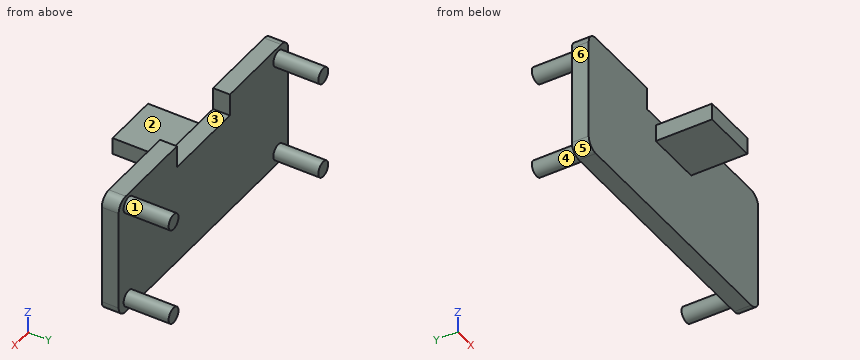
```python
from build123d import *

# Parameters (mm, degrees)
SKETCH1_W           = 48
SKETCH1_H           = 22
BOSS_EXTRUDE1_DEPTH = 3
SKETCH2_R           = 1.4
BOSS_EXTRUDE2_DEPTH = 8
SKETCH3_W           = 10
SKETCH3_H           = 3
BOSS_EXTRUDE3_DEPTH = 10
SKETCH4_W           = 15
SKETCH4_H           = 4
CUT_EXTRUDE1_DEPTH  = 10
FILLET1_R           = 2


with BuildPart() as part:
    # Sketch1 → Boss-Extrude1 (new body)
    with BuildSketch(Plane(origin=(0, 0, 0), x_dir=(1, 0, 0), z_dir=(0, 1, 0))):
        Rectangle(SKETCH1_W, SKETCH1_H)
    extrude(amount=BOSS_EXTRUDE1_DEPTH)

    # Sketch2 → Boss-Extrude2 (add)
    with BuildSketch(Plane(origin=(0, 3, 0), x_dir=(1, 0, 0), z_dir=(0, 1, 0))):
        with Locations((-21.2, 8.899999974)):
            Circle(SKETCH2_R)
        with Locations((-21.2, -8.899999974)):
            Circle(SKETCH2_R)
        with Locations((21.2, 8.899999974)):
            Circle(SKETCH2_R)
        with Locations((21.2, -8.899999974)):
            Circle(SKETCH2_R)
    extrude(amount=BOSS_EXTRUDE2_DEPTH)

    # Sketch3 → Boss-Extrude3 (add)
    with BuildSketch(Plane.XZ):
        with Locations((0, 4.044761195)):
            Rectangle(SKETCH3_W, SKETCH3_H)
    extrude(amount=BOSS_EXTRUDE3_DEPTH)

    # Sketch4 → Cut-Extrude1 (cut)
    with BuildSketch(Plane.XZ):
        with Locations((0, 9)):
            Rectangle(SKETCH4_W, SKETCH4_H)
    extrude(amount=-CUT_EXTRUDE1_DEPTH, mode=Mode.SUBTRACT)

    # Fillet1
    fillet1_edges = [part.edges().sort_by_distance(p)[0] for p in [
        (24, 1.5, 11),
        (-24, 1.5, 11),
        (-24, 1.5, -11),
        (24, 1.5, -11),
    ]]
    fillet(fillet1_edges, radius=FILLET1_R)


solid = part.part
```
Design review of the part built by this model. Coordinates are the model's own, in mm. Face numbers are marked on the shaded views. A direction names the side the tool comes from. Round coordinates to 2 decimals unless told otherwise and drop trailing zeros. Write each loop counter-clockwise with the first axis right and the second up, starting at its lowest first coordinate (ties: lowest second). Pieces come first, ordered by that corner, then holes.
Item 1: We need section A-A on x = 21.2. Write out the cut boundary in (y, z), and give its area (3 significant figures).
Item 2: We need section C-C on z = -8.25. Write out the cut boundary in (x, y), and give its area (3 significant figures).
Item 3: For the marked faces 1, 2 and 3, list the 3-axis set-ups (+Z, -Z, +X, -X, +Y, -Y) from which the entire face can be reached by the end or side of a thin tool; tool diameter is ignored.
Item 4: We need section B-B on y = 6.25. Write out the cut boundary in (x, z).
Item 5: The part is to be moulded in two halves that separate along Z. For the marked faces 4, 5 and 6, say which applies: +Z half, -Z half, draft (parallel to the pull), parting line (faces both ways), or undercut.
Item 6: For probe 1 along X at (y, z) = (9, -8.75); probe 2 along Y at (x, z) = (16, 0); probe 3 along X at (y, z) = (8.25, -9.5), list the stretches that pass through material, from the lowest coordinate up.
Item 7: Clearance check with flat-ended pins moving along their axes: pin 1 Ø2.5 at (y, z) = (-4.5, 3.5) entering from +X; pin 2 Ø1.5 at (x, z) = (-6, -7.5) entering from -Y; pin 3 Ø3 at (x, y) = (2, -5) entering from +Z. State where each tip first meets the part, or that it passes through.
Item 8: We need section D-D on y = -1.25. Write out the cut boundary in (x, z), and give its area (3 significant figures).
Returned:
1. outline: (0, -11) - (3, -11) - (3, -10.3) - (11, -10.3) - (11, -7.5) - (3, -7.5) - (3, 7.5) - (11, 7.5) - (11, 10.3) - (3, 10.3) - (3, 11) - (0, 11) - close
1. area: 111 mm2
2. outline: (-24, 0) - (24, 0) - (24, 3) - (22.44, 3) - (22.44, 11) - (19.96, 11) - (19.96, 3) - (-19.96, 3) - (-19.96, 11) - (-22.44, 11) - (-22.44, 3) - (-24, 3) - close
2. area: 184 mm2
3. face 1: +Y
3. face 2: +Z, +X, -X, -Y
3. face 3: +Z, +Y, -Y
4. outline: circle Ø2.8 at (-21.2, -8.9); circle Ø2.8 at (-21.2, 8.9); circle Ø2.8 at (21.2, -8.9); circle Ø2.8 at (21.2, 8.9)
5. face 4: undercut
5. face 5: -Z half
5. face 6: draft
6. probe 1: x = -22.59 to -19.81, 19.81 to 22.59
6. probe 2: y = 0 to 3
6. probe 3: x = -22.46 to -19.94, 19.94 to 22.46
7. pin 1: stops at x = 5
7. pin 2: stops at y = 0
7. pin 3: stops at z = 5.54
8. outline: (-5, 2.54) - (5, 2.54) - (5, 5.54) - (-5, 5.54) - close
8. area: 30.0 mm2
